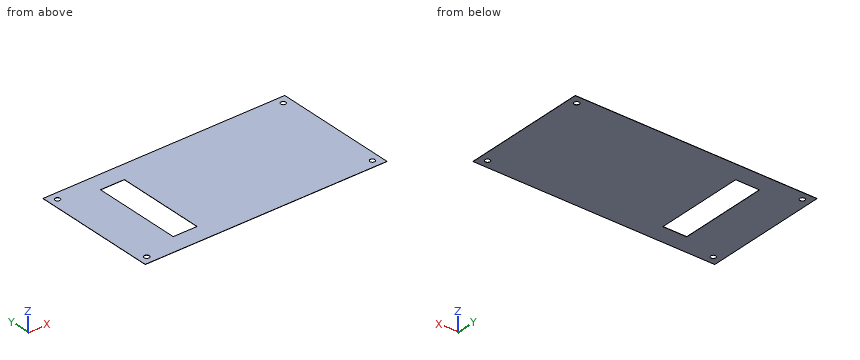
Autodesk Inventor part; units mm, degrees
ref_plane "YZ Plane" through (0, 0, 0) normal (1, 0, 0) x (0, 1, 0)
ref_plane "XZ Plane" through (0, 0, 0) normal (0, 1, 0) x (-1, 0, 0)
ref_plane "XY Plane" through (0, 0, 0) normal (0, 0, 1) x (1, 0, 0)
sketch "Sketch1" plane through (0, 0, 0) normal (0, 0, 1) x (1, 0, 0)
  line L0 (0, 0) -> (145.9, 0)
  line L1 (145.9, 0) -> (145.9, 75.9)
  line L2 (145.9, 75.9) -> (0, 75.9)
  line L3 (0, 75.9) -> (0, 0)
  dimension "d0" = 145.9
  dimension "d1" = 75.9
extrude "Extrusion1" add sketch "Sketch1" along normal blind 0.1
sketch "Sketch2" plane through (0, 0, 0.1) normal (0, 0, 1) x (1, 0, 0)
  line L0 (0, 0) -> (145.9, 0) construction
  line L1 (145.9, 0) -> (145.9, 75.9) construction
  line L2 (145.9, 75.9) -> (0, 75.9) construction
  line L3 (0, 75.9) -> (0, 0) construction
  line L4 (141.05, 4.85) -> (4.85, 4.85) construction
  line L5 (4.85, 4.85) -> (4.85, 71.05) construction
  line L6 (4.85, 71.05) -> (141.05, 71.05) construction
  line L7 (141.05, 71.05) -> (141.05, 4.85) construction
  dimension "d4" = 4.85
hole "Hole1" at (4.85, 71.05, 0.1) at (4.85, 4.85, 0.1) at (141.05, 4.85, 0.1) at (141.05, 71.05, 0.1) direction (0, 0, -1) diameter 3 end through all
sketch "Sketch3" plane through (0, 0, 0.1) normal (0, 0, 1) x (1, 0, 0)
  line L0 (25.8, 10.95) -> (40.2, 10.95)
  line L1 (40.2, 10.95) -> (40.2, 64.95)
  line L2 (40.2, 64.95) -> (25.8, 64.95)
  line L3 (25.8, 64.95) -> (25.8, 10.95)
  circle A0 centre (141.05, 4.85) radius 1.5 construction
  circle A1 centre (4.85, 71.05) radius 1.5 construction
  circle A2 centre (4.85, 4.85) radius 1.5 construction
  circle A3 centre (141.05, 71.05) radius 1.5 construction
  line L4 (0, 0) -> (145.9, 0) construction
  line L5 (145.9, 0) -> (145.9, 75.9) construction
  line L6 (145.9, 75.9) -> (0, 75.9) construction
  line L7 (0, 75.9) -> (0, 0) construction
  dimension "d20" = 105.7
  dimension "d21" = 14.4
  dimension "d22" = 54
  dimension "d23" = 10.95
extrude "Extrusion2" cut sketch "Sketch3" against normal up to next
properties part number "Paper Sheet" material "Paper"
Could you check a few things on this model? Use its own coordinates, in mm. Coordinates: 2 decimals unless noted, no trailing zeros. Write each loop counter-clockwise with the first axis right and the second up, starting at its lowest first coordinate (ties: lowest second). Pieces come first, ordered by that corner, then holes. Notation, with made-up numbers: (40, -17) - (51, -17) arc R13 cw to (51, -11) - close; hole circle Ø9 at (70, -23). An arc over 180 degrees is marked (long way). Write item = value, one per line.
1) Suppose I cut it at B-B on x = 4.85. Please give me the cut outline in (y, z).
Result set:
outline = (0, 0) - (3.35, 0) - (3.35, 0.1) - (0, 0.1) - close; (6.35, 0) - (69.55, 0) - (69.55, 0.1) - (6.35, 0.1) - close; (72.55, 0) - (75.9, 0) - (75.9, 0.1) - (72.55, 0.1) - close
2) Please list where these lines run through material, in increasing order: line 1 (Y direction, x = 37.5, z = 0.05); line 2 (X direction, y = 54, z = 0.05). Write a range as [from, to].
Result set:
line_1 = [0, 10.95], [64.95, 75.9]
line_2 = [0, 25.8], [40.2, 145.9]
3) Suppose I cut it at C-C on y = 40.5. Please give me the cut outline in (x, z), plus the area to 4 significant figures.
Result set:
outline = (0, 0) - (25.8, 0) - (25.8, 0.1) - (0, 0.1) - close; (40.2, 0) - (145.9, 0) - (145.9, 0.1) - (40.2, 0.1) - close
area = 13.15 mm2
4) Will this pin go through, and if not, where does the flat tip stop? pin 1 Ø2.5 at (x, y) = (4.85, 4.85) entering from +Z.
Result set:
pin_1 = through
5) Suppose I cut it at A-A on y = 4.85. Please give me the cut outline in (x, z).
Result set:
outline = (0, 0) - (3.35, 0) - (3.35, 0.1) - (0, 0.1) - close; (6.35, 0) - (139.55, 0) - (139.55, 0.1) - (6.35, 0.1) - close; (142.55, 0) - (145.9, 0) - (145.9, 0.1) - (142.55, 0.1) - close
